Read the model definition and answer for the solid it produces. Units are mm, in the model's axes. A direction names the side the tool comes from. Coordinates: 2 decimals unless noted, no trailing zeros. Write each loop counter-clockwise with the first axis right and the second up, starting at its lowest first coordinate (ties: lowest second). Pieces come first, ordered by that corner, then holes.
(1) Find the intervals of material crossed by probe 1 along Y at (x, z) = (0, 22); probe 2 along Y at (x, z) = (-1, 8.5); probe 3 along X at (y, z) = (1, 15), in increasing order.
(2) Section A-A on z = 21 is taken. Write down the section's boundary in (x, y), then the cut area to 3 significant figures.
(3) Given pin 1 (1.5 mm diameter, centred on y = -35.5, z = 10, fed in from -X); pin 2 (10 mm diameter, centred on x = -17.5, z = 27, fed in from +Y); pin 3 (2 mm diameter, centred on x = 31.81, y = -24.26, fed in from -Z); pin 4 (10 mm diameter, centred on x = -1, z = 5, fed in from -Y), each flat-ended and moving along its own axis, determine where each tip first touches the part or whether it passes through.
(4) The mould has two halves that part along Z. Classify faces 1 (the cylindrical face through (23.1, 31.33, 14.79)), 2 (the flat face through (0, 0, 10)), 3 (the conical face through (9.23, 1.68, 5.18)): +Z half, -Z half, draft (parallel to the pull), parting line (faces both ways), or undercut.
(5) Which of the six approach directions +Z, -Z, +X, -X, +Y, -Y give full straight-line access (tool end or side, diameter ignored) to faces 4 (the conical face through (1.848, -8.942, 5.297)), 5 (the flat face through (-1, 1, 0)), 6 (the cylindrical face through (-29.97, 1.32, 20.14))?
from build123d import *

# Parameters (mm, degrees)
SKIZZE1_R                            = 50
AUFSATZ_LINEAR_AUSTRAGEN1_DEPTH      = 30
SKIZZE2_R                            = 30
SCHNITT_LINEAR_AUSTRAGEN1_DEPTH      = 20
F_3_5_3_5_DURCHMESSER_BOHRUNG1_D     = 3.5
F_3_5_3_5_DURCHMESSER_BOHRUNG1_DEPTH = 40
F_3_5_3_5_DURCHMESSER_BOHRUNG1_TIP   = 1.051506083
F_2_5_2_5_DURCHMESSER_BOHRUNG1_D     = 2.5
F_2_5_2_5_DURCHMESSER_BOHRUNG1_DEPTH = 40
F_2_5_2_5_DURCHMESSER_BOHRUNG1_TIP   = 0.751075774
F_2_0_2_DURCHMESSER_BOHRUNG1_D       = 2
F_2_0_2_DURCHMESSER_BOHRUNG1_DEPTH   = 40
F_2_0_2_DURCHMESSER_BOHRUNG1_TIP     = 0.600860619
F_1_5_1_5_DURCHMESSER_BOHRUNG1_D     = 1.5
F_1_5_1_5_DURCHMESSER_BOHRUNG1_DEPTH = 40
F_1_5_1_5_DURCHMESSER_BOHRUNG1_TIP   = 0.450645464
F_3_5_3_5_DURCHMESSER_BOHRUNG2_D     = 3.5
F_2_5_2_5_DURCHMESSER_BOHRUNG2_D     = 2.5
F_2_0_2_DURCHMESSER_BOHRUNG2_D       = 2
F_1_5_1_5_DURCHMESSER_BOHRUNG3_D     = 1.5


with BuildPart() as part:
    # Skizze1 → Aufsatz-Linear austragen1 (new body)
    with BuildSketch(Plane.XY):
        Circle(SKIZZE1_R)
    extrude(amount=AUFSATZ_LINEAR_AUSTRAGEN1_DEPTH)

    # Skizze2 → Schnitt-Linear austragen1 (cut)
    with BuildSketch(Plane.XY.offset(30)):
        Circle(SKIZZE2_R)
    extrude(amount=-SCHNITT_LINEAR_AUSTRAGEN1_DEPTH, mode=Mode.SUBTRACT)

    # Ø3.5 (3.5) Durchmesser Bohrung1
    with Locations(Plane(origin=(9.764219033, -49.037332989, 5), x_dir=(-0.980746659782, -0.195284380652, 0), z_dir=(0.195284380652, -0.980746659782, 0))):
        with Locations((0, 0)):
            Hole(F_3_5_3_5_DURCHMESSER_BOHRUNG1_D / 2, depth=F_3_5_3_5_DURCHMESSER_BOHRUNG1_DEPTH)
            with Locations((0, 0, -(F_3_5_3_5_DURCHMESSER_BOHRUNG1_DEPTH + F_3_5_3_5_DURCHMESSER_BOHRUNG1_TIP / 2))):  # 118° drill point
                Cone(0, F_3_5_3_5_DURCHMESSER_BOHRUNG1_D / 2, F_3_5_3_5_DURCHMESSER_BOHRUNG1_TIP, mode=Mode.SUBTRACT)

    # Ø2.5 (2.5) Durchmesser Bohrung1
    with Locations(Plane(origin=(49.30181814, 8.326507554, 5), x_dir=(-0.166530151078, 0.986036362809, 0), z_dir=(0.986036362809, 0.166530151078, 0))):
        with Locations((0, 0)):
            Hole(F_2_5_2_5_DURCHMESSER_BOHRUNG1_D / 2, depth=F_2_5_2_5_DURCHMESSER_BOHRUNG1_DEPTH)
            with Locations((0, 0, -(F_2_5_2_5_DURCHMESSER_BOHRUNG1_DEPTH + F_2_5_2_5_DURCHMESSER_BOHRUNG1_TIP / 2))):  # 118° drill point
                Cone(0, F_2_5_2_5_DURCHMESSER_BOHRUNG1_D / 2, F_2_5_2_5_DURCHMESSER_BOHRUNG1_TIP, mode=Mode.SUBTRACT)

    # Ø2.0 (2) Durchmesser Bohrung1
    with Locations(Plane(origin=(-9.221972092, 49.142193996, 5), x_dir=(0.982843879919, 0.184439441837, 0), z_dir=(-0.184439441837, 0.982843879919, 0))):
        with Locations((0, 0)):
            Hole(F_2_0_2_DURCHMESSER_BOHRUNG1_D / 2, depth=F_2_0_2_DURCHMESSER_BOHRUNG1_DEPTH)
            with Locations((0, 0, -(F_2_0_2_DURCHMESSER_BOHRUNG1_DEPTH + F_2_0_2_DURCHMESSER_BOHRUNG1_TIP / 2))):  # 118° drill point
                Cone(0, F_2_0_2_DURCHMESSER_BOHRUNG1_D / 2, F_2_0_2_DURCHMESSER_BOHRUNG1_TIP, mode=Mode.SUBTRACT)

    # Ø1.5 (1.5) Durchmesser Bohrung1
    with Locations(Plane(origin=(-48.958569775, -10.151770565, 5), x_dir=(0.203035411308, -0.979171395495, 0), z_dir=(-0.979171395495, -0.203035411308, 0))):
        with Locations((0, 0)):
            Hole(F_1_5_1_5_DURCHMESSER_BOHRUNG1_D / 2, depth=F_1_5_1_5_DURCHMESSER_BOHRUNG1_DEPTH)
            with Locations((0, 0, -(F_1_5_1_5_DURCHMESSER_BOHRUNG1_DEPTH + F_1_5_1_5_DURCHMESSER_BOHRUNG1_TIP / 2))):  # 118° drill point
                Cone(0, F_1_5_1_5_DURCHMESSER_BOHRUNG1_D / 2, F_1_5_1_5_DURCHMESSER_BOHRUNG1_TIP, mode=Mode.SUBTRACT)

    # Ø3.5 (3.5) Durchmesser Bohrung2 (through all)
    with Locations(Plane.XY.offset(30)):
        with Locations((31.806649029, -24.255660732)):
            Hole(F_3_5_3_5_DURCHMESSER_BOHRUNG2_D / 2)

    # Ø2.5 (2.5) Durchmesser Bohrung2 (through all)
    with Locations(Plane.XY.offset(30)):
        with Locations((24.254021663, 31.807898911)):
            Hole(F_2_5_2_5_DURCHMESSER_BOHRUNG2_D / 2)

    # Ø2.0 (2) Durchmesser Bohrung2 (through all)
    with Locations(Plane.XY.offset(30)):
        with Locations((-31.809148709, 24.25238253)):
            Hole(F_2_0_2_DURCHMESSER_BOHRUNG2_D / 2)

    # Ø1.5 (1.5) Durchmesser Bohrung3 (through all)
    with Locations(Plane.XY.offset(30)):
        with Locations((-24.250743333, -31.810398422)):
            Hole(F_1_5_1_5_DURCHMESSER_BOHRUNG3_D / 2)


solid = part.part
Response:
1. probe 1: y = -50 to -30, 30 to 50
1. probe 2: y = -49.99 to 49.99
1. probe 3: x = -49.99 to -29.98, 29.98 to 49.99
2. outline: circle Ø100 at (0, 0); hole circle Ø2 at (-31.81, 24.25); hole circle Ø60 at (0, 0); hole circle Ø1.5 at (-24.25, -31.81); hole circle Ø2.5 at (24.25, 31.81); hole circle Ø3.5 at (31.81, -24.26)
2. area: 5,010 mm2
3. pin 1: stops at x = -35.95
3. pin 2: stops at y = 48.41
3. pin 3: passes through
3. pin 4: stops at y = -50
4. face 1: draft
4. face 2: +Z half
4. face 3: undercut
5. face 4: none
5. face 5: -Z, +X, -X, +Y, -Y
5. face 6: +Z
